The listing builds one solid part. Answer for the finished solid, in the listing's coordinates (mm). A direction names the side the tool comes from. Round coordinates to 2 decimals unless told otherwise and drop trailing zeros. Write each loop counter-clockwise with the first axis right and the second up, starting at its lowest first coordinate (ties: lowest second). Pieces come first, ordered by that corner, then holes. Notation, with made-up numbers: (14.25, 74) - (35.25, 74) arc R18 cw to (35.25, 93) - close; hole circle Ø8 at (81.5, 44). An arc over 180 degrees is marked (long way). Return JSON: item names as keys, results as strings. Group by question number.
from build123d import *

# Parameters (mm, degrees)
F0_W      = 30
F0_H      = 30
F1_DEPTH  = 35
F2_W      = 40
F2_H      = 40
F3_DEPTH  = 20
F4_SIZE   = 18
F5_R      = 8.1403588374
F6_DEPTH  = 20
F7_R      = 2.5
F8_DEPTH  = 7.5
F9_R      = 2.5
F10_DEPTH = 79.502
F11_W     = 5
F11_H     = 5
F12_DEPTH = 15
F13_R     = 10
F13_R_2   = 5
F14_DEPTH = 2.5


# Not quite as in the source:
# - a feature names something its author has since deleted; it is built from what else it names


with BuildPart() as f1:
    # F0 (on Top) → F1 (new body)
    with BuildSketch(Plane.XY):
        Rectangle(F0_W, F0_H)
    extrude(amount=F1_DEPTH)

    # F2 (on face) → F3 (join)
    with BuildSketch(Plane.XY.offset(35)):
        Rectangle(F2_W, F2_H)
    extrude(amount=F3_DEPTH)

    # F4
    f4_edges = [f1.edges().sort_by_distance(p)[0] for p in [
        (20, 0, 55),
        (0, 20, 55),
        (-20, 0, 55),
        (0, -20, 55),
    ]]
    chamfer(f4_edges, length=F4_SIZE)

    # F5 (on face) → F6 (cut)
    with BuildSketch(Plane.YZ.offset(15)):
        with Locations((0, 23.1403588374)):
            Circle(F5_R)
    extrude(amount=-F6_DEPTH, mode=Mode.SUBTRACT)

    # F7 (on face) → F8 (join)
    with BuildSketch(Plane.YZ.offset(15)):
        with Locations((0, 7.5)):
            Circle(F7_R)
    extrude(amount=F8_DEPTH)

    # F9 (on face) → F10 (cut)
    with BuildSketch(Plane.YZ.offset(20)):
        with Locations((0, 50)):
            Circle(F9_R)
    extrude(amount=-F10_DEPTH, mode=Mode.SUBTRACT)

    # F11 (on face) → F12 (join)
    with BuildSketch(Plane(origin=(0, 0, 0), x_dir=(1, 0, 0), z_dir=(0, 0, -1))):
        Rectangle(F11_W, F11_H)
    extrude(amount=F12_DEPTH)

    # F13 (on Right) → F14 (join, symmetric)
    with BuildSketch(Plane.YZ):
        with Locations((0, -20)):
            Circle(F13_R)
        with Locations((0, -20)):
            Circle(F13_R_2, mode=Mode.SUBTRACT)
    extrude(amount=F14_DEPTH, both=True)


solid = f1.part
(1) Consider line 1 (Z direction, x = 1, y = 0); line 2 (Z direction, x = 5, y = 0); line 3 (Y direction, x = 0, z = -20). Determine where each line is inside the solid, lowest interval first.
(2) For faces 1 (the flat face through (0, -2.5, -5)), 2 (the flat face through (-15, 0, 17)), 3 (the flat face through (0, 15, 17)), determine the directions among +Z, -Z, +X, -X, +Y, -Y from which every point of the face is accessible in a straight line to the end or side of a thin tool.
(3) Find section C-C (x = -12). Write down the section's boundary in (y, z), plus the area to 3 significant figures.
(4) Determine the mould class of faces 4 (the cylindrical face through (0.13, -0.54, 47.56)), 5 (the flat face through (2.5, -0.1, -14.8)), 6 (the flat face through (0, 13, 44)) for opening direction Z: +Z half, -Z half, draft (parallel to the pull), parting line (faces both ways), or undercut.
(5) Flat-ended cylindrical pins translate along their axes: pin 1 (10 mm diameter, centred on y = 13.5, z = 28, fed in from +X); pin 2 (10 mm diameter, centred on x = -13, z = 22, fed in from +Y); pin 3 (11.5 mm diameter, centred on y = 0, z = -20, fed in from +X). Find the tip coordinate at first contact, or state that the pin passes through.
(6) Find section A-A (z = 50). Write down the section's boundary in (x, y), plus the area to 3 significant figures.
(7) Find section B-B (y = 0). State how many separate pieces and enclosed holes the cut face has, plus the area to 3 significant figures.
(8) Find section D-D (z = 7.5). Write down the section's boundary in (x, y).
Check sheet entries:
{
 "1": {"line 1": "z = -30 to -25, -15 to 15, 31.28 to 47.5, 52.5 to 55", "line 2": "z = 0 to 15, 31.28 to 47.5", "line 3": "y = -10 to -5, 5 to 10"},
 "2": {"face 1": "+X, -X, -Y", "face 2": "-Z, -X, +Y, -Y", "face 3": "-Z, +X, -X, +Y"},
 "3": {"outline": "(-20, 35) - (-15, 35) - (-15, 0) - (15, 0) - (15, 35) - (20, 35) - (20, 37) - (12, 45) - (-12, 45) - (-20, 37) - close", "area": "1,390 mm^2"},
 "4": {"face 4": "undercut", "face 5": "draft", "face 6": "+Z half"},
 "5": {"pin 1": "stops at x = 15", "pin 2": "stops at y = 15", "pin 3": "stops at x = 2.5"},
 "6": {"outline": "(-7, -7) - (7, -7) - (7, -2.5) - (-7, -2.5) - close; (-7, 2.5) - (7, 2.5) - (7, 7) - (-7, 7) - close", "area": "126 mm^2"},
 "7": {"separate pieces": "3", "enclosed holes": "0", "area": "1,270 mm^2"},
 "8": {"outline": "(-15, -15) - (15, -15) - (15, -2.5) - (22.5, -2.5) - (22.5, 2.5) - (15, 2.5) - (15, 15) - (-15, 15) - close"}
}
